from build123d import *

# Parameters (mm, degrees)
BOSS_EXTRU_1_DEPTH = 92.5
ESQUISSE2_R        = 16.1
ESQUISSE2_R_2      = 1.7
ESQUISSE2_R_3      = 9.6
BOSS_EXTRU_2_DEPTH = 2.2


with BuildPart() as part:
    # Esquisse1 → Boss.-Extru.1 (new body, symmetric)
    with BuildSketch(Plane.XY):
        with BuildLine():
            Line((-25, 0), (-25, -37.200306763))
            Line((-25, -37.200306763), (25, -37.200306763))
            Line((25, -37.200306763), (25, 0))
            Line((25, 0), (16.1, 0))
            ThreePointArc((16.1, 0), (0, -16.1), (-16.1, 0))
            Line((-16.1, 0), (-25, 0))
        make_face()
    extrude(amount=BOSS_EXTRU_1_DEPTH, both=True)

    # Esquisse2 → Boss.-Extru.2 (add)
    with BuildSketch(Plane.XY.offset(92.5)):
        Circle(ESQUISSE2_R)
        with Locations((0, 13)):
            Circle(ESQUISSE2_R_2, mode=Mode.SUBTRACT)
        Circle(ESQUISSE2_R_3, mode=Mode.SUBTRACT)
        with Locations((9.192388155, 9.192388155)):
            Circle(ESQUISSE2_R_2, mode=Mode.SUBTRACT)
        with Locations((13, 0)):
            Circle(ESQUISSE2_R_2, mode=Mode.SUBTRACT)
        with Locations((9.192388155, -9.192388155)):
            Circle(ESQUISSE2_R_2, mode=Mode.SUBTRACT)
        with Locations((0, -13)):
            Circle(ESQUISSE2_R_2, mode=Mode.SUBTRACT)
        with Locations((-9.192388155, -9.192388155)):
            Circle(ESQUISSE2_R_2, mode=Mode.SUBTRACT)
        with Locations((-13, 0)):
            Circle(ESQUISSE2_R_2, mode=Mode.SUBTRACT)
        with Locations((-9.192388155, 9.192388155)):
            Circle(ESQUISSE2_R_2, mode=Mode.SUBTRACT)
    boss_extru_2 = extrude(amount=-BOSS_EXTRU_2_DEPTH)

    # Symétrie1: Boss.-Extru.2 across plane
    add(boss_extru_2.mirror(Plane.XY))


solid = part.part
The model under review builds one solid part; all positions refer to its coordinate system, in mm. A direction names the side the tool comes from. Round coordinates to 2 decimals unless told otherwise and drop trailing zeros. Write each loop counter-clockwise with the first axis right and the second up, starting at its lowest first coordinate (ties: lowest second). Pieces come first, ordered by that corner, then holes. Notation, with made-up numbers: M 56,-20.75 L 66,-20.75 A12 cw 66,-8.75 Z; hole C -25.75,-8 d11. An arc over 180 degrees is marked long. Answer as CSV lines item,"result". Start each with the question number.
Q1. Consider section A-A, the plane y = -3.5. Give the boundary of the cut face in (x, z), then the cut area to 3 significant figures.
Q2. Consider section B-B, the plane x = 13. Give the boundary of the cut face in (y, z).
Q3. The part is to be moulded in two halves that separate along Y. For faces 3 (the face through (0, -16, 92.5)), 4 (the face through (21, 0, 1)), 5 (the face through (-0.221, -11.314, 91.415)), say which applies: +Y half, -Y half, draft (parallel to the pull), parting line (faces both ways), or undercut.
Q4. Wall thickness on line 1 along Y through (x, z) = (0, -92); line 2 along Z through (x, y) = (-12, 5.5); line 3 along Y through (x, z) = (-1, -44): over which ranges is each line inside the solid? List them lowest first.
Q5. Consider section D-D, the plane y = 13. Give the boundary of the cut face in (x, z), then the cut area to 3 significant figures.
Q6. Tool access review of faces 1 (the face through (7, -7, -90.3)), 2 (the face through (0.354, 16.096, 91.415)): name each direction out of +Z, -Z, +X, -X, +Y, -Y from which nothing blocks a thin tool from reaching the whole face with its end or side.
Q7. Consider section C-C, the plane z = 71. Give the boundary of the cut face in (x, y).
Q8. Clearance check with flat-ended pins moving along their axes: P1, Ø10, axis at y = 6.5, z = 70, coming from the +X side; P2, Ø1.5, axis at x = -15.5, z = 13.5, coming from the +Y side. State where each tip first meets the part, or that it passes through.
Result set:
1,outline,"M -25,-92.5 L -8.94,-92.5 L -8.94,-90.3 L -15.71,-90.3 L -15.71,90.3 L -8.94,90.3 L -8.94,92.5 L -25,92.5 Z; M 8.94,-92.5 L 25,-92.5 L 25,92.5 L 8.94,92.5 L 8.94,90.3 L 15.71,90.3 L 15.71,-90.3 L 8.94,-90.3 Z"
1,area,"3,500 mm²"
2,outline,"M -37.2,-92.5 L -1.7,-92.5 L -1.7,-90.3 L -9.5,-90.3 L -9.5,90.3 L -1.7,90.3 L -1.7,92.5 L -37.2,92.5 Z; M 1.7,-92.5 L 9.5,-92.5 L 9.5,-90.3 L 1.7,-90.3 Z; M 1.7,90.3 L 9.5,90.3 L 9.5,92.5 L 1.7,92.5 Z"
3,face 3,"draft"
3,face 4,"+Y half"
3,face 5,"undercut"
4,line 1,"y = -37.2 to -14.7, -11.3 to -9.6, 9.6 to 11.3, 14.7 to 16.1"
4,line 2,"z = -92.5 to -90.3, 90.3 to 92.5"
4,line 3,"y = -37.2 to -16.07"
5,outline,"M -9.5,-92.5 L -1.7,-92.5 L -1.7,-90.3 L -9.5,-90.3 Z; M -9.5,90.3 L -1.7,90.3 L -1.7,92.5 L -9.5,92.5 Z; M 1.7,-92.5 L 9.5,-92.5 L 9.5,-90.3 L 1.7,-90.3 Z; M 1.7,90.3 L 9.5,90.3 L 9.5,92.5 L 1.7,92.5 Z"
5,area,"68.6 mm²"
6,face 1,"+Y"
6,face 2,"+Z, -Z, +Y"
7,outline,"M -25,-37.2 L 25,-37.2 L 25,0 L 16.1,0 A16.1 cw -16.1,0 L -25,0 Z"
8,P1,"passes through"
8,P2,"stops at y = 0"
